Answer from the drawing. Dimensions are ordinates in mm from the lowest x, y and z of the part. A direction names the side the tool comes from. Give positions to 0.01 mm unless a question says otherwise; leave off trailing zeros. Write each loop counter-clockwise with the first axis right and the second up, starting at its lowest first coordinate (ties: lowest second). Pieces come first, ordered by that corner, then holes.
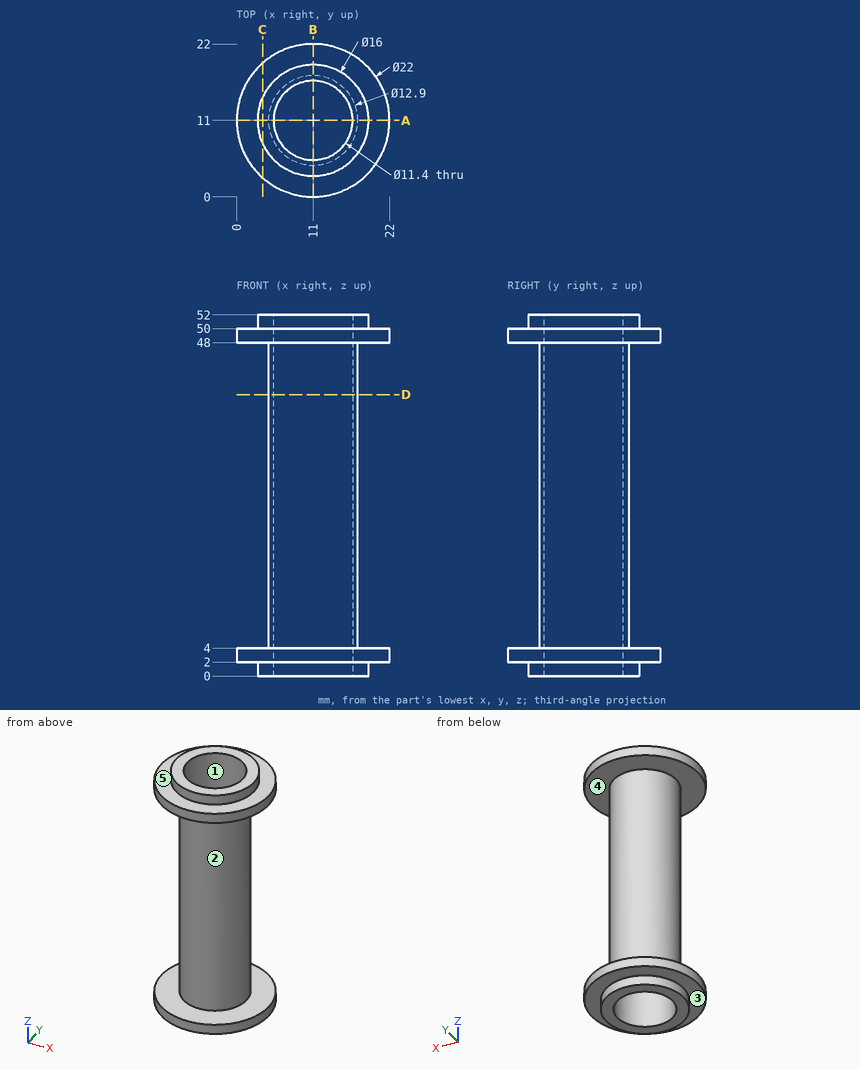
Item 1: A cutting plane is placed at C-C, the plane x = 3.75. Give the vertices of the cut face in (y, z), plus the area to 3 significant figures.
Conclusion:
outline: (2.73, 2) - (7.62, 2) - (7.62, 0) - (14.38, 0) - (14.38, 2) - (19.27, 2) - (19.27, 4) - (2.73, 4) - close; (2.73, 48) - (19.27, 48) - (19.27, 50) - (14.38, 50) - (14.38, 52) - (7.62, 52) - (7.62, 50) - (2.73, 50) - close
area: 93.2 mm2
Item 2: Consider probe 1 along Z at (x, y) = (6, 20.25); probe 2 along Y at (x, z) = (11, 30); probe 3 along Z at (x, y) = (18, 12.75). Determine where each line is inside the solid, lowest interval first.
Conclusion:
probe 1: z = 2 to 4, 48 to 50
probe 2: y = 4.55 to 5.3, 16.7 to 17.45
probe 3: z = 0 to 4, 48 to 52
Item 3: A cutting plane is placed at D-D, the plane z = 40.5. Give the vertices of the cut face in (x, y).
Conclusion:
outline: circle Ø12.9 at (11, 11); hole circle Ø11.4 at (11, 11)
Item 4: A cutting plane is placed at A-A, the plane y = 11. Give the vertices of the cut face in (x, z).
Conclusion:
outline: (0, 2) - (3, 2) - (3, 0) - (5.3, 0) - (5.3, 52) - (3, 52) - (3, 50) - (0, 50) - (0, 48) - (4.55, 48) - (4.55, 4) - (0, 4) - close; (16.7, 0) - (19, 0) - (19, 2) - (22, 2) - (22, 4) - (17.45, 4) - (17.45, 48) - (22, 48) - (22, 50) - (19, 50) - (19, 52) - (16.7, 52) - close
Item 5: Each of these flat-tipped pins is pushed along its axis until it touches: P1, Ø8, axis at x = 18, z = 15, coming from the -Y side; P2, Ø8, axis at y = 11.5, z = 18, coming from the -X side; P3, Ø1, axis at x = 5, z = 38.5, coming from the +Y side. Where does it stop, or does it pass through?
Conclusion:
P1: stops at y = 5.29
P2: stops at x = 4.55
P3: stops at y = 14.37
Item 6: Which of the six approach directions +Z, -Z, +X, -X, +Y, -Y give full straight-line access (tool end or side, diameter ignored) to the marked faces 4 and 5?
Conclusion:
face 4: none
face 5: +Z
Item 7: Determine the mould class of the marked faces 1, 2 and 3 for opening direction X: pulls with the +X half, pulls with the -X half, needs draft (parallel to the pull), parting line crosses it, or undercut.
Conclusion:
face 1: undercut
face 2: parting line crosses it
face 3: needs draft
